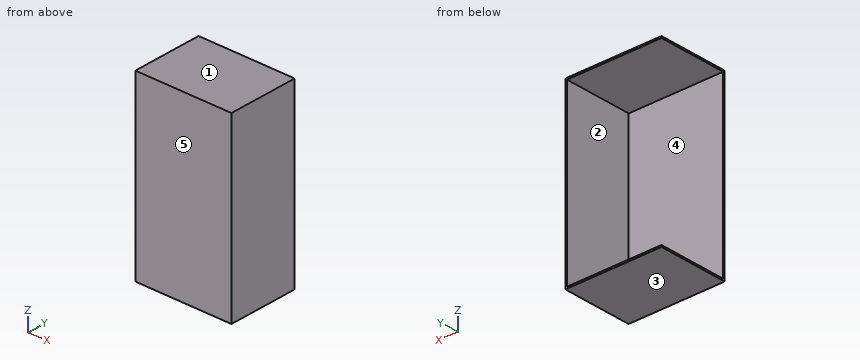
Autodesk Inventor part; units mm, degrees
ref_plane "YZ Plane" through (0, 0, 0) normal (1, 0, 0) x (0, 1, 0)
ref_plane "XZ Plane" through (0, 0, 0) normal (0, 1, 0) x (-1, 0, 0)
ref_plane "XY Plane" through (0, 0, 0) normal (0, 0, 1) x (1, 0, 0)
sketch "Sketch1" plane through (0, 0, 0) normal (0, 1, 0) x (-1, 0, 0)
  line L0 (0, 0) -> (-177.8, 0)
  line L1 (-177.8, 0) -> (-177.8, -333.375)
  line L2 (-177.8, -333.375) -> (0, -333.375)
  line L3 (0, -333.375) -> (0, 0)
  dimension "d0" = 177.8
  dimension "d1" = 333.375
extrude "Extrusion1" add sketch "Sketch1" along normal blind 3.175
sketch "Sketch2" plane through (0, 3.175, 0) normal (0, 1, 0) x (1, 0, 0)
  line L0 (0, 333.375) -> (0, 0) construction
  line L1 (0, 3.175) -> (174.625, 3.175)
  line L2 (174.625, 3.175) -> (174.625, 330.2)
  line L3 (174.625, 330.2) -> (0, 330.2)
  line L4 (177.8, 333.375) -> (0, 333.375)
  line L5 (177.8, 0) -> (177.8, 333.375)
  line L6 (0, 0) -> (177.8, 0)
  line L7 (0, 0) -> (0, 3.175)
  line L8 (0, 330.2) -> (0, 333.375)
  dimension "d4" = 3.175
  dimension "d5" = 3.175
  dimension "d6" = 3.175
extrude "Extrusion2" add sketch "Sketch2" along normal blind 127
Geometry check sheet. Reference: the model listing, model coordinates, mm. Face numbers are marked on the shaded views. A direction names the side the tool comes from. Round coordinates to 2 decimals unless told otherwise and drop trailing zeros. Order: outer loops, then holes, each group sorted by start corner. A loop starts at its lowest first (then second) coordinate and runs counter-clockwise, first axis right, second up. Notation, with made-up numbers: (67, -34) - (118, -34) arc R23 cw to (118, -20) - close; hole circle Ø7 at (62.5, 86.25). An arc over 180 degrees is marked (long way). Use a Markdown table: item, result. Add a question column.
1) Set-up check for the marked faces 1 and 2: record each of +Z, -Z, +X, -X, +Y, -Y from which the full face is reachable in a straight line by a thin tool's end or side.
2) Section check A-A (x = 90.5). Record the cut outline in (y, z) (3 decimals), then the cut area to 3 significant figures.
3) Section check B-B (y = 57.5). Record the cut outline in (x, z) (3 decimals).
4) Gauge pin test, flat ends, axial feed: P1, Ø1, axis at x = 150, y = 35, coming from the +Z side; P2, Ø1.5, axis at x = 89, z = -73.5, coming from the +Y side (3 decimals). Record the tip position at first contact, or that the pin passes through.
5) Thickness scan on line 1 along Z through (x, y) = (106, 76) (3 decimals); line 2 along X through (y, z) = (102.5, -99) (3 decimals); line 3 along Y through (x, z) = (161, -130) (3 decimals). Record the ranges inside material, lowest first.
6) Section check C-C (z = -72). Record the cut outline in (x, y) (3 decimals), then the cut area to 3 significant figures.
7) Mould release check, pull along Z, two halves, no side actions. Record for the marked faces 3, 4 and 5: released by +Z, released by -Z, zero draft, split by the parting line, or undercut.
Established:
| question | item | result |
|---|---|---|
| 1 | face 1 | +Z, +X, -X, +Y, -Y |
| 1 | face 2 | -X, +Y |
| 2 | outline | (0, -333.375) - (130.175, -333.375) - (130.175, -330.2) - (3.175, -330.2) - (3.175, -3.175) - (130.175, -3.175) - (130.175, 0) - (0, 0) - close |
| 2 | area | 1,860 mm2 |
| 3 | outline | (0, -333.375) - (177.8, -333.375) - (177.8, 0) - (0, 0) - (0, -3.175) - (174.625, -3.175) - (174.625, -330.2) - (0, -330.2) - close |
| 4 | P1 | z = 0 |
| 4 | P2 | y = 3.175 |
| 5 | line 1 | -333.375 to -330.2, -3.175 to 0 |
| 5 | line 2 | 174.625 to 177.8 |
| 5 | line 3 | 0 to 3.175 |
| 6 | outline | (0, 0) - (177.8, 0) - (177.8, 130.175) - (174.625, 130.175) - (174.625, 3.175) - (0, 3.175) - close |
| 6 | area | 968 mm2 |
| 7 | face 3 | released by -Z |
| 7 | face 4 | undercut |
| 7 | face 5 | zero draft |
